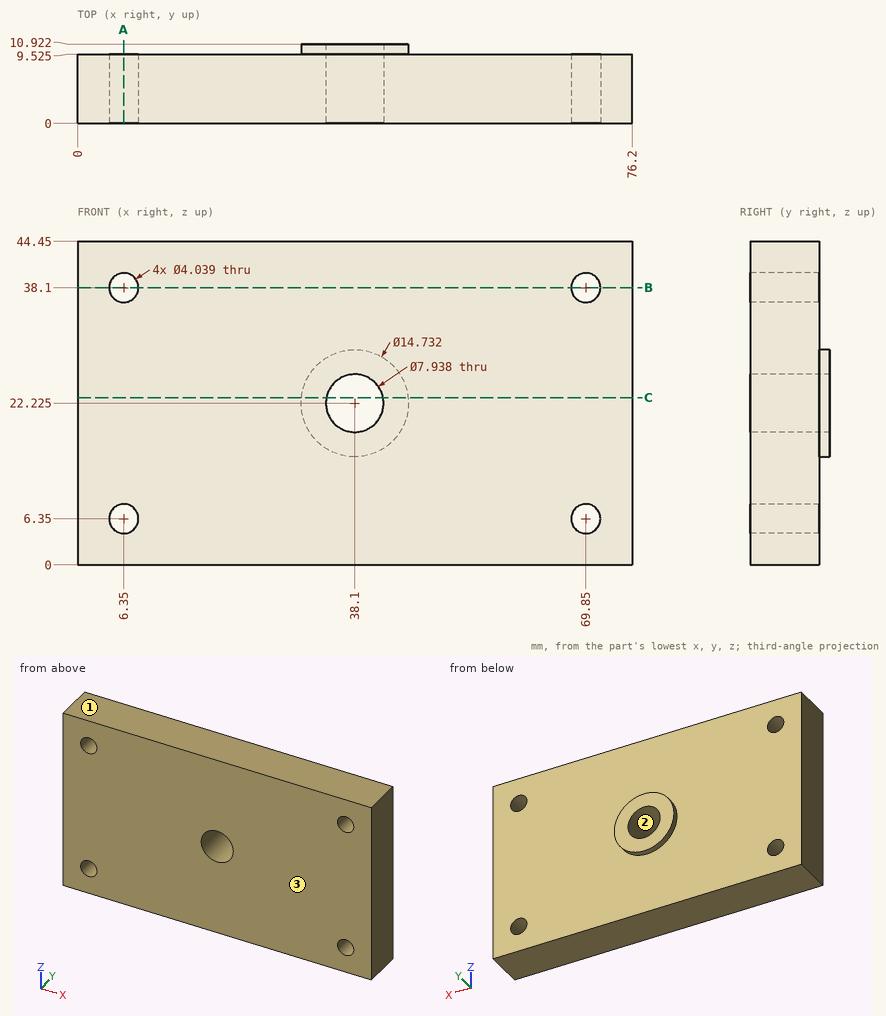
Study the drawing (mm; zero at the part's minimum x, y, z) and answer. Coordinates: 2 decimals unless noted, no trailing zeros. Write each loop counter-clockwise with the first axis right and the second up, starting at its lowest first coordinate (ties: lowest second). Pieces come first, ordered by that corner, then holes. Notation, with made-up numbers: (67.5, 82) - (99.5, 82) arc R32 cw to (99.5, 116) - close; hole circle Ø5 at (29, 61). An arc over 180 degrees is marked (long way). Put each result on its own line as item: value.
1. Flat-ended cylindrical pins translate along their axes: pin 1 Ø6.5 at (x, z) = (38.1, 22.225) entering from -Y; pin 2 Ø2 at (x, z) = (9.5, 30) entering from +Y (1 decimal). Find the tip coordinate at first contact, or state that the pin passes through.
Answer sheet:
pin 1: passes through
pin 2: stops at y = 9.5
2. The part is cut by section B-B on z = 38.1. Give the vertices of the cut face in (x, y) (1 decimal), plus the area to 3 significant figures.
Answer sheet:
outline: (0, 0) - (4.3, 0) - (4.3, 9.5) - (0, 9.5) - close; (8.4, 0) - (67.8, 0) - (67.8, 9.5) - (8.4, 9.5) - close; (71.9, 0) - (76.2, 0) - (76.2, 9.5) - (71.9, 9.5) - close
area: 649 mm^2
3. Find the intervals of material crossed by line 1 along Z through (x, y) = (69.85, 5.25); line 2 along Y through (x, z) = (53.5, 9) (1 decimal); line 3 along Z through (x, y) = (38.1, 6.5), in increasing order. Write a range as from..to.
Answer sheet:
line 1: z = 0..4.33, 8.37..36.08, 40.12..44.45
line 2: y = 0..9.5
line 3: z = 0..18.26, 26.19..44.45
4. The part is cut by section A-A on x = 6.35. State how many separate pieces and enclosed holes the cut face has.
Answer sheet:
separate pieces: 3
enclosed holes: 0
5. Determine the mould class of the marked faces 1, 2 and 3 for opening direction Z: pulls with the +Z half, pulls with the -Z half, needs draft (parallel to the pull), parting line crosses it, or undercut.
Answer sheet:
face 1: pulls with the +Z half
face 2: undercut
face 3: needs draft
6. The part is cut by section C-C on z = 23. Give the vertices of the cut face in (x, y) (1 decimal), plus the area to 3 significant figures.
Answer sheet:
outline: (0, 0) - (34.2, 0) - (34.2, 10.9) - (30.8, 10.9) - (30.8, 9.5) - (0, 9.5) - close; (42, 0) - (76.2, 0) - (76.2, 9.5) - (45.4, 9.5) - (45.4, 10.9) - (42, 10.9) - close
area: 661 mm^2
